```python
from build123d import *

# Parameters (mm, degrees)
SKETCH1_W                      = 80.3
SKETCH1_H                      = 66
BOSS_EXTRUDE1_DEPTH            = 2
F_3_2_3_2_DIAMETER_HOLE1_D     = 3.2
FILLET1_R                      = 3
SKETCH4_W                      = 80.3
SKETCH4_H                      = 2
BOSS_EXTRUDE2_DEPTH            = 42
FILLET2_R                      = 20
F_3_2_3_2_DIAMETER_HOLE2_D     = 3.2
F_3_2_3_2_DIAMETER_HOLE2_DEPTH = 60
F_3_2_3_2_DIAMETER_HOLE2_TIP   = 0.96137699


with BuildPart() as part:
    # Sketch1 → Boss-Extrude1 (new body)
    with BuildSketch(Plane.XY):
        with Locations((40.15, 33)):
            Rectangle(SKETCH1_W, SKETCH1_H)
    extrude(amount=BOSS_EXTRUDE1_DEPTH)

    # Ø3.2 (3.2) Diameter Hole1 (through all)
    with Locations(Plane.XY.offset(2)):
        with Locations((7, 59), (73.3, 59), (73.3, 7), (7, 7)):
            Hole(F_3_2_3_2_DIAMETER_HOLE1_D / 2)

    # Fillet1
    fillet1_edges = [part.edges().sort_by_distance(p)[0] for p in [
        (0, 66, 1),
        (80.3, 66, 1),
    ]]
    fillet(fillet1_edges, radius=FILLET1_R)

    # Sketch4 → Boss-Extrude2 (add)
    with BuildSketch(Plane.XZ):
        with Locations((40.15, 1)):
            Rectangle(SKETCH4_W, SKETCH4_H)
    extrude(amount=BOSS_EXTRUDE2_DEPTH)

    # Fillet2
    fillet2_edges = [part.edges().sort_by_distance(p)[0] for p in [
        (0, -42, 1),
        (80.3, -42, 1),
    ]]
    fillet(fillet2_edges, radius=FILLET2_R)

    # Ø3.2 (3.2) Diameter Hole2
    with Locations(Plane.XY.offset(2)):
        with Locations((7, -27), (73.3, -27)):
            Hole(F_3_2_3_2_DIAMETER_HOLE2_D / 2, depth=F_3_2_3_2_DIAMETER_HOLE2_DEPTH)
            with Locations((0, 0, -(F_3_2_3_2_DIAMETER_HOLE2_DEPTH + F_3_2_3_2_DIAMETER_HOLE2_TIP / 2))):  # 118° drill point
                Cone(0, F_3_2_3_2_DIAMETER_HOLE2_D / 2, F_3_2_3_2_DIAMETER_HOLE2_TIP, mode=Mode.SUBTRACT)


solid = part.part
```
Geometry check sheet. Reference: the model listing, model coordinates, mm. Coordinates: 2 decimals unless noted, no trailing zeros. Order: outer loops, then holes, each group sorted by start corner. A loop starts at its lowest first (then second) coordinate and runs counter-clockwise, first axis right, second up. Notation, with made-up numbers: (88, 3) - (125, 3) arc R24 ccw to (125, 18) - close; hole circle Ø9 at (-26, 36). An arc over 180 degrees is marked (long way). Answer as a JSON object with one key per item and string values. Group by question number.
Item 1: Sectioned sample at B-B, the plane z = 1.4. Record the cut outline in (x, y).
Item 2: Depth check by flat-ended pin: pin 1 Ø1 at (x, z) = (16.5, 1) entering from -Y. Enter the tip coordinate at first touch or a pass-through.
Item 3: Sectioned sample at D-D, the plane y = -27. Record the cut outline in (x, z).
Item 4: Scan lines: probe 1 along Y at (x, z) = (7, 0.7); probe 2 along X at (y, z) = (-23, 0.25); probe 3 along Y at (x, z) = (4.5, 1.8). Record each from-to range of solid material in increasing order.
Item 5: Sectioned sample at A-A, the plane y = 59. Record the cut outline in (x, z), and give its area (3 significant figures).
Item 6: Draft check along X on faces 1 (the face through (74.9, -26.93, 0.99)), 2 (the face through (40, 13, 0)), 3 (the face through (5.703, -35.986, 1.014)), 4 (the face through (74.597, -35.986, 1.014)). Enter one of: +X half, -X half, draft (parallel to the pull), parting line (faces both ways), or undercut.
Item 7: Sectioned sample at C-C, the plane x = 73.3. Record the cut outline in (y, z), and give its area (3 significant figures).
Resolved:
{
 "1": {"outline": "(0, -22) arc R20 ccw to (20, -42) - (60.3, -42) arc R20 ccw to (80.3, -22) - (80.3, 63) arc R3 ccw to (77.3, 66) - (3, 66) arc R3 ccw to (0, 63) - close; hole circle Ø3.2 at (7, -27); hole circle Ø3.2 at (7, 7); hole circle Ø3.2 at (7, 59); hole circle Ø3.2 at (73.3, -27); hole circle Ø3.2 at (73.3, 7); hole circle Ø3.2 at (73.3, 59)"},
 "2": {"pin 1": "y = -41.77"},
 "3": {"outline": "(0.64, 0) - (5.4, 0) - (5.4, 2) - (0.64, 2) - close; (8.6, 0) - (71.7, 0) - (71.7, 2) - (8.6, 2) - close; (74.9, 0) - (79.66, 0) - (79.66, 2) - (74.9, 2) - close"},
 "4": {"probe 1": "-37.2 to -28.6, -25.4 to 5.4, 8.6 to 57.4, 60.6 to 66", "probe 2": "0.03 to 80.27", "probe 3": "-34.64 to 66"},
 "5": {"outline": "(0, 0) - (5.4, 0) - (5.4, 2) - (0, 2) - close; (8.6, 0) - (71.7, 0) - (71.7, 2) - (8.6, 2) - close; (74.9, 0) - (80.3, 0) - (80.3, 2) - (74.9, 2) - close", "area": "148 mm^2"},
 "6": {"face 1": "undercut", "face 2": "draft", "face 3": "-X half", "face 4": "+X half"},
 "7": {"outline": "(-37.2, 0) - (-28.6, 0) - (-28.6, 2) - (-37.2, 2) - close; (-25.4, 0) - (5.4, 0) - (5.4, 2) - (-25.4, 2) - close; (8.6, 0) - (57.4, 0) - (57.4, 2) - (8.6, 2) - close; (60.6, 0) - (66, 0) - (66, 2) - (60.6, 2) - close", "area": "187 mm^2"}
}
